```python
from build123d import *

# Parameters (mm, degrees)
SKETCH1_R           = 6.5
BOSS_EXTRUDE1_DEPTH = 3
SKETCH2_R           = 5.5
FILLET1_R           = 2
SKETCH3_R           = 0.5
CUT_EXTRUDE1_DEPTH  = 0.5
SKETCH4_R           = 5
CUT_EXTRUDE2_DEPTH  = 1.8
SKETCH5_W           = 1.5
SKETCH5_H           = 3.5
SKETCH5_W_2         = 1.7
SKETCH5_H_2         = 1.5
BOSS_EXTRUDE3_DEPTH = 5
BOSS_EXTRUDE4_DEPTH = 3.5
FILLET2_R           = 1


with BuildPart() as part:
    # Sketch1 → Boss-Extrude1 (new body)
    with BuildSketch(Plane(origin=(0, 0, 0), x_dir=(1, 0, 0), z_dir=(0, 1, 0))):
        Circle(SKETCH1_R)
    extrude(amount=BOSS_EXTRUDE1_DEPTH)

    # Sketch2 → section 0 of loft1
    with BuildSketch(Plane(origin=(0, 6, 0), x_dir=(1, 0, 0), z_dir=(0, 1, 0)), mode=Mode.PRIVATE) as loft1_s0:
        Circle(SKETCH2_R)
    # loft up to a face of the part (loft1)
    loft([loft1_s0.sketch, part.faces().sort_by_distance((0, 3, 0))[0]])

    # Fillet1
    fillet1_edges = [part.edges().sort_by_distance(p)[0] for p in [
        (-5.5, 6, 0),
    ]]
    fillet(fillet1_edges, radius=FILLET1_R)

    # Sketch3 → Cut-Extrude1 (cut)
    with BuildSketch(Plane(origin=(0, 6, 0), x_dir=(1, 0, 0), z_dir=(0, 1, 0))):
        with BuildLine():
            Line((0.5, 0), (0.5, 3.435004881))
            ThreePointArc((0.5, 3.435004881), (0, 3.935004881), (-0.5, 3.435004881))
            Line((-0.5, 3.435004881), (-0.5, 0))
            ThreePointArc((-0.5, 0), (0, -0.5), (0.5, 0))
        make_face()
        with BuildLine():
            ThreePointArc((-1.408185783, 1.802395609), (-2.110021897, 1.888570248), (-2.023847258, 2.590406363))
            ThreePointArc((-2.023847258, 2.590406363), (0, -3.287272859), (2.023847258, 2.590406363))
            ThreePointArc((2.023847258, 2.590406363), (2.165413544, 2.415586559), (2.21601652, 2.196400986))
            ThreePointArc((2.21601652, 2.196400986), (1.935202094, 1.747003963), (1.408185783, 1.802395609))
            ThreePointArc((1.408185783, 1.802395609), (0, -2.287272859), (-1.408185783, 1.802395609))
        make_face()
        with Locations((1.71601652, 2.196400986)):
            Circle(SKETCH3_R)
        with Locations((-1.71601652, 2.196400986)):
            Circle(SKETCH3_R)
    extrude(amount=-CUT_EXTRUDE1_DEPTH, mode=Mode.SUBTRACT)

    # Sketch4 → Cut-Extrude2 (cut)
    with BuildSketch(Plane.XZ):
        Circle(SKETCH4_R)
    extrude(amount=-CUT_EXTRUDE2_DEPTH, mode=Mode.SUBTRACT)

    # Sketch5 → Boss-Extrude3 (add)
    with BuildSketch(Plane.XZ.offset(-1.8)):
        with Locations((2.5, 0)):
            Rectangle(SKETCH5_W, SKETCH5_H)
        with Locations((0, -2.5)):
            Rectangle(SKETCH5_W_2, SKETCH5_H_2)
        with Locations((-2.5, 0)):
            Rectangle(SKETCH5_W, SKETCH5_H)
        with Locations((0, 2.5)):
            Rectangle(SKETCH5_W_2, SKETCH5_H_2)
    extrude(amount=BOSS_EXTRUDE3_DEPTH)

    # Sketch6 → Boss-Extrude4 (add)
    with BuildSketch(Plane.XY.offset(1.75)):
        Polygon((1.75, -3.2), (1, -2.5), (1.75, -2.5), align=None)
    boss_extrude4 = extrude(amount=-BOSS_EXTRUDE4_DEPTH)

    # Mirror1: Boss-Extrude4 across plane
    add(boss_extrude4.mirror(Plane(origin=(0, 0, 0), x_dir=(0, 0, 1), z_dir=(1, 0, 0))))

    # Fillet2
    fillet2_edges = [part.edges().sort_by_distance(p)[0] for p in [
        (3.25, 1.8, 0),
        (0, 1.8, -3.25),
        (-3.25, 1.8, 0),
        (0, 1.8, 3.25),
    ]]
    fillet(fillet2_edges, radius=FILLET2_R)


solid = part.part
```
Model file for the job. Use its own axes, mm. A direction names the side the tool comes from. Coordinates: 2 decimals unless noted, no trailing zeros. Loops run counter-clockwise (first coordinate to the right, second up) from the corner with the lowest first, then second, coordinate; pieces in that order, holes last. Notation, with made-up numbers: (-38, 52.25) - (-2, 52.25) arc R22 ccw to (-2, 65.25) - close; hole circle Ø5 at (19, 64.25). An arc over 180 degrees is marked (long way). Write item = value, one per line. Start each with the question number.
Item 1: Saw through at C-C, the plane y = 5. List the corners of the cut face in (x, z).
Item 2: Saw through at A-A, the plane y = -1.75. List the corners of the cut face in (x, z), then the cut area to 3 significant figures.
Item 3: 3-axis set-ups, long thin cutter, end or side, ignore diameter. For faces 3 (the face through (1.75, 0, 0)), 4 (the face through (2, -3.2, 0)), 5 (the face through (0.079, 5.754, 2.286)), 6 (the face through (-0.85, -1, 2)): which of +Z, -Z, +X, -X, +Y, -Y reach the whole face in a straight line?
Item 4: Pull direction X, two halves, no side cores. Call faces 1 (the face through (2, 0, 5)), 2 (the face through (0, 1.8, 0)): +X half, -X half, draft (parallel to the pull), parting line (faces both ways), or undercut.
Item 5: Drop flat-ended pins along their axis: pin 1 Ø1.9 at (x, y) = (0.5, -1) entering from +Z; pin 2 Ø3 at (x, y) = (2.5, 0) entering from +Z; pin 3 Ø1.5 at (y, z) = (3.5, -1.5) entering from +X; pin 4 Ø4 at (x, z) = (-0.5, 4.5) entering from -Y. Give the stop position or say it passes through.
Item 6: Wall check: probe 1 along X at (y, z) = (-1, 1.5); probe 2 along Z at (x, y) = (0, 1.15); probe 3 along Y at (x, z) = (-3, 2.75). Give the ranges that are in metal, low to high. Write a range as [from, to].
Answers:
q1.outline = circle Ø11.58 at (0, 0)
q2.outline = (-3.25, -1.75) - (-1.75, -1.75) - (-1.75, 1.75) - (-3.25, 1.75) - close; (-0.85, -3.25) - (0.85, -3.25) - (0.85, -1.75) - (-0.85, -1.75) - close; (-0.85, 1.75) - (0.85, 1.75) - (0.85, 3.25) - (-0.85, 3.25) - close; (1.75, -1.75) - (3.25, -1.75) - (3.25, 1.75) - (1.75, 1.75) - close
q2.area = 15.6 mm2
q3.face_3 = none
q3.face_4 = +Z, -Z, +X, -X, -Y
q3.face_5 = +Y
q3.face_6 = -Y
q4.face_1 = draft
q4.face_2 = undercut
q5.pin_1 = 3.25
q5.pin_2 = 6.42
q5.pin_3 = 6.43
q5.pin_4 = -3.2
q6.probe_1 = [-3.25, -1.75], [1.75, 3.25]
q6.probe_2 = [-6.5, -5], [-3.31, -1.75], [1.75, 3.31], [5, 6.5]
q6.probe_3 = [1.8, 6]
